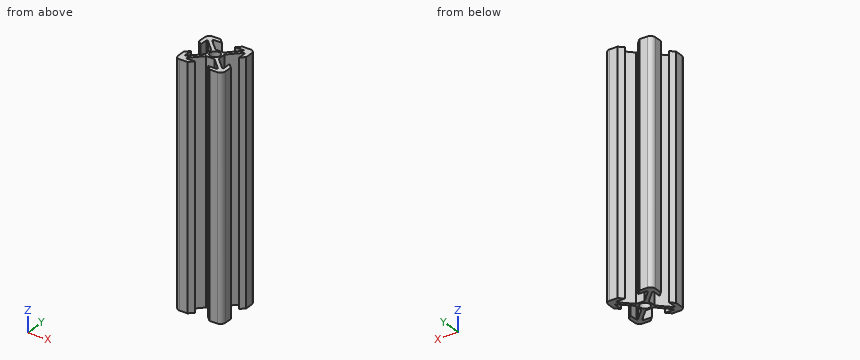
from build123d import *

# Parameters (mm, degrees)
SKETCH1_W           = 5.68
SKETCH1_H           = 5.68
SKETCH1_R           = 2.1
BOSS_EXTRUDE1_DEPTH = 100


with BuildPart() as part:
    # Sketch1 → Boss-Extrude1 (new body)
    with BuildSketch(Plane.XY):
        Rectangle(SKETCH1_W, SKETCH1_H)
        Circle(SKETCH1_R, mode=Mode.SUBTRACT)
        with BuildLine():
            ThreePointArc((-10, 8), (-9.414213562, 9.414213562), (-8, 10))
            Line((-8, 10), (-4.64, 10))
            Line((-4.64, 10), (-2.84, 8.2))
            Line((-2.84, 8.2), (-6.56, 8.2))
            Line((-6.56, 8.2), (-6.56, 6.56))
            Line((-6.56, 6.56), (-8.2, 6.56))
            Line((-8.2, 6.56), (-8.2, 2.84))
            Line((-8.2, 2.84), (-10, 4.64))
            Line((-10, 4.64), (-10, 8))
        make_face()
        with BuildLine():
            Line((10, 4.64), (10, 8))
            ThreePointArc((10, 8), (9.414213562, 9.414213562), (8, 10))
            Line((8, 10), (4.64, 10))
            Line((4.64, 10), (2.84, 8.2))
            Line((2.84, 8.2), (6.56, 8.2))
            Line((6.56, 8.2), (6.56, 6.56))
            Line((6.56, 6.56), (8.2, 6.56))
            Line((8.2, 6.56), (8.2, 2.84))
            Line((8.2, 2.84), (10, 4.64))
        make_face()
        with BuildLine():
            Line((-10, -4.64), (-10, -8))
            ThreePointArc((-10, -8), (-9.414213562, -9.414213562), (-8, -10))
            Line((-8, -10), (-4.64, -10))
            Line((-4.64, -10), (-2.84, -8.2))
            Line((-2.84, -8.2), (-6.56, -8.2))
            Line((-6.56, -8.2), (-6.56, -6.56))
            Line((-6.56, -6.56), (-8.2, -6.56))
            Line((-8.2, -6.56), (-8.2, -2.84))
            Line((-8.2, -2.84), (-10, -4.64))
        make_face()
        with BuildLine():
            Line((4.64, -10), (8, -10))
            ThreePointArc((8, -10), (9.414213562, -9.414213562), (10, -8))
            Line((10, -8), (10, -4.64))
            Line((10, -4.64), (8.2, -2.84))
            Line((8.2, -2.84), (8.2, -6.56))
            Line((8.2, -6.56), (6.56, -6.56))
            Line((6.56, -6.56), (6.56, -8.2))
            Line((6.56, -8.2), (2.84, -8.2))
            Line((2.84, -8.2), (4.64, -10))
        make_face()
        Polygon((7.620660172, -6.56), (2.84, -1.779339828), (2.84, -2.84), (6.56, -6.56), align=None)
        Polygon((6.56, -6.56), (2.84, -2.84), (1.779339828, -2.84), (6.56, -7.620660172), align=None)
        Polygon((-1.779339828, -2.84), (-2.84, -2.84), (-6.56, -6.56), (-6.56, -7.620660172), align=None)
        Polygon((-2.84, -2.84), (-2.84, -1.779339828), (-7.620660172, -6.56), (-6.56, -6.56), align=None)
        Polygon((-2.84, 1.779339828), (-2.84, 2.84), (-6.56, 6.56), (-7.620660172, 6.56), align=None)
        Polygon((-2.84, 2.84), (-1.779339828, 2.84), (-6.56, 7.620660172), (-6.56, 6.56), align=None)
        Polygon((6.56, 6.56), (6.56, 7.620660172), (1.779339828, 2.84), (2.84, 2.84), align=None)
        Polygon((7.620660172, 6.56), (6.56, 6.56), (2.84, 2.84), (2.84, 1.779339828), align=None)
    extrude(amount=BOSS_EXTRUDE1_DEPTH)


solid = part.part
Could you check a few things on this model? Use its own coordinates, in mm. Give positions to 0.01 mm unless a question says otherwise; leave off trailing zeros. Order: outer loops, then holes, each group sorted by start corner. A loop starts at its lowest first (then second) coordinate and runs counter-clockwise, first axis right, second up. Notation, with made-up numbers: (41.5, 19.5) - (76.5, 19.5) arc R19 cw to (76.5, 34.5) - close; hole circle Ø8 at (11, -7). An arc over 180 degrees is marked (long way). Return JSON: item names as keys, results as strings. Group by question number.
Q1. Please list where these lines run through material, in increasing order: line 1 along Y through (x, z) = (0, 38); line 2 along X through (y, z) = (-6.25, 76.5); line 3 along X through (y, z) = (-8, 40). Write a range as [from, to].
Q2. Will these pins go through, and if not, where does the flat tip stop? pin 1 Ø1.8 at (y, z) = (-0.5, 59.5) entering from +X; pin 2 Ø3 at (x, y) = (4, -6) entering from +Z; pin 3 Ø5 at (x, z) = (0.5, 76) entering from +Y; pin 4 Ø1.1 at (y, z) = (-4, 42.5) entering from +X.
Q3. Suppose I cut it at A-A, the plane y = 0. Please give me the cut outline in (x, z), and give its area (3 significant figures).
Resolved:
{
 "1": {"line 1": "y = [-2.84, -2.1], [2.1, 2.84]", "line 2": "x = [-10, -8.2], [-7.31, -5.19], [5.19, 7.31], [8.2, 10]", "line 3": "x = [-10, -6.56], [6.56, 10]"},
 "2": {"pin 1": "stops at x = 2.84", "pin 2": "stops at z = 100", "pin 3": "stops at y = 8.36", "pin 4": "stops at x = 9.91"},
 "3": {"outline": "(-2.84, 0) - (-2.1, 0) - (-2.1, 100) - (-2.84, 100) - close; (2.1, 0) - (2.84, 0) - (2.84, 100) - (2.1, 100) - close", "area": "148 mm2"}
}
